Design review of the part built by this model. Coordinates are the model's own, in mm. Face numbers are marked on the shaded views. A direction names the side the tool comes from. Give positions to 0.01 mm unless a question says otherwise; leave off trailing zeros. Write each loop counter-clockwise with the first axis right and the second up, starting at its lowest first coordinate (ties: lowest second). Pieces come first, ordered by that corner, then holes. Notation, with made-up numbers: M -21,89.5 L 32,89.5 A11 cw 32,106.5 Z; hole C 31,-1 d3. An arc over 180 degrees is marked long. Answer in a Markdown table with one row per item.
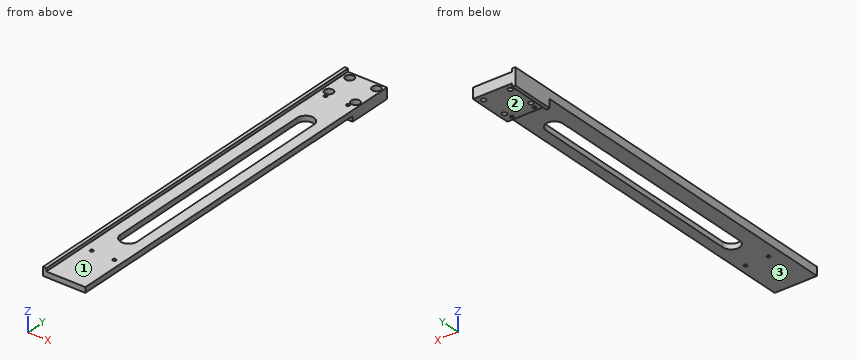
```python
from build123d import *

# Parameters (mm, degrees)
SKETCH1_W                      = 30
SKETCH1_H                      = 290.3
BOSS_EXTRUDE1_DEPTH            = 8
SKETCH1_3_W                    = 2.5
SKETCH1_3_H                    = 290.3
BOSS_EXTRUDE2_DEPTH            = 10.35
SKETCH1_6_W                    = 2.5
SKETCH1_6_H                    = 290.3
BOSS_EXTRUDE3_DEPTH            = 2.35
CBORE_FOR_M3_SHCS1_D           = 3.6
CBORE_FOR_M3_SHCS1_CBORE_D     = 6.5
CBORE_FOR_M3_SHCS1_CBORE_DEPTH = 4
M3X0_5_TAPPED_HOLE1_D          = 2.5
CUT_EXTRUDE1_DEPTH             = 10
SKETCH12_W                     = 0.75
SKETCH12_H                     = 290.3
CUT_EXTRUDE2_DEPTH             = 147.567032446
SKETCH15_W                     = 31.75
SKETCH15_H                     = 257.3
CUT_EXTRUDE3_DEPTH             = 4
CUT_EXTRUDE3_DIRECTION_2_REACH = 148.567


with BuildPart() as part:
    # Sketch1 → Boss-Extrude1 (new body)
    with BuildSketch(Plane.XY):
        Rectangle(SKETCH1_W, SKETCH1_H)
    extrude(amount=BOSS_EXTRUDE1_DEPTH)

    # Sketch1<3> → Boss-Extrude2 (add)
    with BuildSketch(Plane.XY):
        with Locations((-16.25, 0)):
            Rectangle(SKETCH1_3_W, SKETCH1_3_H)
    extrude(amount=BOSS_EXTRUDE2_DEPTH)

    # Sketch1<6> → Boss-Extrude3 (add)
    with BuildSketch(Plane.XY):
        with Locations((-16.25, 0)):
            Rectangle(SKETCH1_6_W, SKETCH1_6_H)
    extrude(amount=-BOSS_EXTRUDE3_DEPTH)

    # CBORE for M3 SHCS1 (through all)
    with Locations(Plane.XY.offset(8)):
        with Locations((-10, 140.35), (10, 140.35), (10, 120.35), (-10, 120.35)):
            CounterBoreHole(CBORE_FOR_M3_SHCS1_D / 2, CBORE_FOR_M3_SHCS1_CBORE_D / 2, CBORE_FOR_M3_SHCS1_CBORE_DEPTH)

    # M3x0.5 Tapped Hole1 (through all)
    with Locations(Plane.XY.offset(8)):
        with Locations((-8.5, 115.15), (8.5, 115.15), (8.5, -109.85), (-8.5, -109.85)):
            Hole(M3X0_5_TAPPED_HOLE1_D / 2)

    # Sketch11 → Cut-Extrude1 (cut)
    with BuildSketch(Plane.XY.offset(8)):
        with BuildLine():
            Line((-6.35, -85), (-6.35, 85))
            ThreePointArc((-6.35, 85), (0, 91.35), (6.35, 85))
            Line((6.35, 85), (6.35, -85))
            ThreePointArc((6.35, -85), (0, -91.35), (-6.35, -85))
        make_face()
    extrude(amount=-CUT_EXTRUDE1_DEPTH, mode=Mode.SUBTRACT)

    # Sketch12 → Cut-Extrude2 (cut, through all)
    with BuildSketch(Plane.XY.offset(8)):
        with Locations((14.625, 0)):
            Rectangle(SKETCH12_W, SKETCH12_H)
    extrude(amount=-CUT_EXTRUDE2_DEPTH, mode=Mode.SUBTRACT)

    # Sketch15 → Cut-Extrude3 (cut)
    with BuildSketch(Plane(origin=(0, 0, 0), x_dir=(-1, 0, 0), z_dir=(0, 0, -1))):
        with Locations((1.625, -16.5)):
            Rectangle(SKETCH15_W, SKETCH15_H)
    extrude(amount=-CUT_EXTRUDE3_DEPTH, mode=Mode.SUBTRACT)

    # Cut-Extrude3 direction 2: up to this face of the body (flat: up to its plane)
    cut_extrude3_direction_2_end = Plane(part.part.faces().sort_by_distance((-16.25, 0, -2.35))[0])
    # Sketch15 → Cut-Extrude3 direction 2 (cut, up to the picked face)
    with BuildSketch(Plane(origin=(0, 0, 0), x_dir=(-1, 0, 0), z_dir=(0, 0, -1)), mode=Mode.PRIVATE) as cut_extrude3_direction_2_sk1:
        with Locations((1.625, -16.5)):
            Rectangle(SKETCH15_W, SKETCH15_H)
    cut_extrude3_direction_2_tool1 = split(extrude(cut_extrude3_direction_2_sk1.sketch, amount=CUT_EXTRUDE3_DIRECTION_2_REACH, mode=Mode.PRIVATE), bisect_by=cut_extrude3_direction_2_end, keep=Keep.BOTH, mode=Mode.PRIVATE)
    add(cut_extrude3_direction_2_tool1.solids().sort_by(Axis((-1.625, -16.5, 0), (0, 0, -1)))[0], mode=Mode.SUBTRACT)


solid = part.part
```
1) To check wall thickness, follow probe 1 along Y at (x, z) = (10, 2.85); probe 2 along X at (y, z) = (140.35, 4.8); probe 3 along Y at (x, z) = (10, 5.75). State the ranges of each line that lie inside material, in increasing order. Write a range as [from, to].
Geometry says:
| item | result |
|---|---|
| probe 1 | [112.15, 118.55], [122.15, 138.55], [142.15, 145.15] |
| probe 2 | [-17.5, -13.25], [-6.75, 6.75], [13.25, 14.25] |
| probe 3 | [-145.15, 117.1], [123.6, 137.1], [143.6, 145.15] |
2) Insertion check: P1, Ø3, axis at x = 8.5, y = -109.85, coming from the +Z side; P2, Ø4, axis at x = 10, y = 120.35, coming from the -Z side; P3, Ø2, axis at x = -9.5, y = 121.5, coming from the +Z side; P4, Ø3, axis at x = -10, y = 140.35, coming from the -Z side. Each pin has a flat end and moves straight along its axis. Give the tip position at first contact, or say it passes through.
Geometry says:
| item | result |
|---|---|
| P1 | z = 8 |
| P2 | z = 0 |
| P3 | z = 4 |
| P4 | through |
3) For the marked faces 1, 2 and 3, list the 3-axis set-ups (+Z, -Z, +X, -X, +Y, -Y) from which the entire face can be reached by the end or side of a thin tool; tool diameter is ignored.
Geometry says:
| item | result |
|---|---|
| face 1 | +Z, +X, +Y, -Y |
| face 2 | -Z, +X, +Y, -Y |
| face 3 | -Z, +X, -X, -Y |
4) Add section A-A (y = 41.5). Write out the cut boundary in (x, z), and give its area (3 significant figures).
Geometry says:
| item | result |
|---|---|
| outline | M -17.5,4 L -6.35,4 L -6.35,8 L -15,8 L -15,10.35 L -17.5,10.35 Z; M 6.35,4 L 14.25,4 L 14.25,8 L 6.35,8 Z |
| area | 82.1 mm^2 |
